```python
from build123d import *

# Parameters (mm, degrees)
CHAMFER2_SIZE                  = 0.4
CHAMFER2_SIZE2                 = 1.492820323
CHAMFER2_PART_2_SIZE           = 0.4
CHAMFER2_PART_2_SIZE2          = 1.492820323
CBORE_FOR_M5_SBHCS1_AT_2_COUNT = 2
CBORE_FOR_M5_SBHCS1_AT_2_PITCH = 32.5
CBORE_FOR_M5_SBHCS1_AT_3_COUNT = 2
CBORE_FOR_M5_SBHCS1_AT_3_PITCH = 29.455003079
SKETCH16_R                     = 5.55
CUT_EXTRUDE6_DEPTH             = 23
F_2_4_2_4_DIAMETER_HOLE1_D     = 2.4
F_2_4_2_4_DIAMETER_HOLE1_DEPTH = 2
CHAMFER1_SIZE                  = 0.25
CHAMFER1_SIZE2                 = 0.686869355
CUT_EXTRUDE8_DEPTH             = 6.5
FILLET1_R                      = 30


with BuildPart() as part:
    # Sketch1 → Revolve1 (revolve)
    with BuildSketch(Plane.XY):
        Polygon((5, -22), (5, -13), (13.4, -13), (13.4, 0), (23.75, 0), (23.75, 30), (0, 30), (0, -22), align=None)
    revolve(axis=Axis((0, 0, 0), (0, 1, 0)))

    # Chamfer2
    chamfer2_edges = [part.edges().sort_by_distance(p)[0] for p in [
        (-5, -22, 0),
    ]]
    chamfer2_side = [part.faces().sort_by_distance(p)[0] for p in [
        (0, -22, 0),
    ]]
    chamfer(chamfer2_edges, length=CHAMFER2_SIZE, length2=CHAMFER2_SIZE2, reference=chamfer2_side[0])

    # Chamfer2 part 2
    chamfer2_part_2_edges = [part.edges().sort_by_distance(p)[0] for p in [
        (-13.4, -13, 0),
    ]]
    chamfer2_part_2_side = [part.faces().sort_by_distance(p)[0] for p in [
        (-5.379009235, -13, 0),
    ]]
    chamfer(chamfer2_part_2_edges, length=CHAMFER2_PART_2_SIZE, length2=CHAMFER2_PART_2_SIZE2, reference=chamfer2_part_2_side[0])

    # Sketch15 → CBORE for M5 SBHCS1 (revolve, cut)
    with BuildSketch(Plane(origin=(0, 0, 16.25), x_dir=(0, 0, -1), z_dir=(1, 0, 0))):
        Polygon((0, 0), (0, 30), (2.6, 30), (2.6, 24), (5.55, 24), (5.55, 0), align=None)
    cbore_for_m5_sbhcs1 = revolve(axis=Axis((0, -6.35, 16.25), (0, 1, 0)), mode=Mode.SUBTRACT)

    # CBORE for M5 SBHCS1 at 2: CBORE for M5 SBHCS1 ×2
    with Locations(*[(0, 0, -i * CBORE_FOR_M5_SBHCS1_AT_2_PITCH) for i in range(1, CBORE_FOR_M5_SBHCS1_AT_2_COUNT)]):
        add(cbore_for_m5_sbhcs1, mode=Mode.SUBTRACT)

    # CBORE for M5 SBHCS1 at 3: CBORE for M5 SBHCS1 ×2
    with Locations(*[Vector(0.422618262, 0, -0.906307787) * (i * CBORE_FOR_M5_SBHCS1_AT_3_PITCH) for i in range(1, CBORE_FOR_M5_SBHCS1_AT_3_COUNT)]):
        add(cbore_for_m5_sbhcs1, mode=Mode.SUBTRACT)

    # Sketch16 → Cut-Extrude6 (cut, through all)
    with BuildSketch(Plane.XZ):
        with Locations((0, -16.25)):
            Circle(SKETCH16_R)
        with Locations((12.448222201, -10.445298657)):
            Circle(SKETCH16_R)
        with Locations((0, 16.25)):
            Circle(SKETCH16_R)
    extrude(amount=CUT_EXTRUDE6_DEPTH, mode=Mode.SUBTRACT)

    # Ø2.4 (2.4) Diameter Hole1
    with Locations(Plane(origin=(0, 30, 0), x_dir=(1, 0, 0), z_dir=(0, 1, 0))):
        with Locations((0, 21), (16.086933305, 13.498539803), (0, -21)):
            Hole(F_2_4_2_4_DIAMETER_HOLE1_D / 2, depth=F_2_4_2_4_DIAMETER_HOLE1_DEPTH)

    # Chamfer1
    chamfer1_edges = [part.edges().sort_by_distance(p)[0] for p in [
        (1.2, 30, 21),
        (17.286933305, 30, -13.498539803),
        (1.2, 30, -21),
    ]]
    chamfer1_side = [part.faces().sort_by_distance(p)[0] for p in [
        (-0.198929798, 30, 0.16692192),
    ]]
    chamfer(chamfer1_edges, length=CHAMFER1_SIZE, length2=CHAMFER1_SIZE2, reference=chamfer1_side[0])

    # Sketch30 → Cut-Extrude8 (cut, symmetric)
    with BuildSketch(Plane.XY):
        Polygon((-23.75, 30), (23.75, 30), (23.75, 23.504038846), (12.5, 28.75), (-12.5, 28.75), (-23.75, 23.504038846), align=None)
    extrude(amount=CUT_EXTRUDE8_DEPTH, both=True, mode=Mode.SUBTRACT)

    # Fillet1
    fillet1_edges = [part.edges().sort_by_distance(p)[0] for p in [
        (12.5, 28.75, 0),
        (-12.5, 28.75, 0),
    ]]
    fillet(fillet1_edges, radius=FILLET1_R)


solid = part.part
```
CAD build for the part. Positions are in the model's coordinates, mm. A direction names the side the tool comes from. Coordinates: 2 decimals unless noted, no trailing zeros. Order: outer loops, then holes, each group sorted by start corner. A loop starts at its lowest first (then second) coordinate and runs counter-clockwise, first axis right, second up.
(1) Mould opens along Z. For faces 6 (the face through (21.939, 15.21, 9.096)), 7 (the face through (0, -22, 0)), 8 (the face through (-0.78, 26.96, -18.73)) say: released by +Z, released by -Z, zero draft, split by the parting line, or undercut.
Solution:
face 6: split by the parting line
face 7: zero draft
face 8: undercut
(2) Which spindle directions (+Z, -Z, +X, -X, +Y, -Y) get a long thin tool onto all of the face, cutting with end or side? Do faces 1 (the face through (-1.08, -16.7, 4.88)), 2 (the face through (0.26, 28.65, -19.83)), 3 (the face through (-0.78, 26.96, 13.77)), 4 (the face through (5.601, -12.243, -11.956)), 5 (the face through (-12.43, 28.02, 0.09)). Say none if no direction does.
Solution:
face 1: -Y
face 2: +Y
face 3: +Y, -Y
face 4: -Z, +X, -Y
face 5: -X, +Y
(3) Drill centre lines: L1, parallel to Z at x = 0, y = 7.25; L2, parallel to Z at x = 0, y = 27; L3, parallel to X at y = -3.5, z = -0.5. Where is each one in solid material? Low to high.
Solution:
L1: z = -23.75 to -21.8, -10.7 to 10.7, 21.8 to 23.75
L2: z = -23.75 to -18.85, -13.65 to 13.65, 18.85 to 23.75
L3: x = -13.39 to 13.39
(4) Pin check, flat tips, straight feed: pin 1 Ø13 at (x, z) = (0, -16.25) entering from +Y; pin 2 Ø5.5 at (x, z) = (-1.5, -17.5) entering from -Y; pin 3 Ø0.7 at (x, z) = (-0.5, -21.5) entering from +Y; pin 4 Ø3 at (y, z) = (11.5, 11.5) entering from +X. Stop position of each tip, or through.
Solution:
pin 1: stops at y = 30
pin 2: stops at y = 24
pin 3: stops at y = 28
pin 4: stops at x = 21.54
(5) Saw through at B-B, the plane y = -2.5. Write the cut outline in (x, z).
Solution:
outline: (-4.27, -12.7) arc R5.55 cw to (4.27, -12.7) arc R13.4 ccw to (6.99, -11.43) arc R5.55 cw to (12.47, -4.9) arc R13.4 ccw to (4.27, 12.7) arc R5.55 cw to (-4.27, 12.7) arc R13.4 ccw to start
(6) Saw through at A-A, the plane z = 16.25. Write the cut outline in (x, y).
Solution:
outline: (-17.32, 0) - (-5.55, 0) - (-5.55, 24) - (-2.6, 24) - (-2.6, 30) - (-17.32, 30) - close; (2.6, 24) - (5.55, 24) - (5.55, 0) - (17.32, 0) - (17.32, 30) - (2.6, 30) - close
(7) Saw through at C-C, the plane x = 21.5. Write the cut outline in (y, z), and give its area (3 significant figures).
Solution:
outline: (0, -10.09) - (30, -10.09) - (30, -6.5) - (24.55, -6.5) - (24.55, 6.5) - (30, 6.5) - (30, 10.09) - (0, 10.09) - close
area: 535 mm2
(8) Saw through at D-D, the plane z = -21. Write the cut outline in (x, y).
Solution:
outline: (-11.09, 0) - (-2.87, 0) - (-2.87, 24) - (2.87, 24) - (2.87, 0) - (11.09, 0) - (11.09, 30) - (1.45, 30) - (1.2, 29.31) - (1.2, 28) - (-1.2, 28) - (-1.2, 29.31) - (-1.45, 30) - (-11.09, 30) - close
